The listing builds one solid part. Answer for the finished solid, in the listing's coordinates (mm). Coordinates: 2 decimals unless noted, no trailing zeros. Order: outer loops, then holes, each group sorted by start corner. A loop starts at its lowest first (then second) coordinate and runs counter-clockwise, first axis right, second up. Notation, with made-up numbers: (45, 43.5) -> (61, 43.5) arc R16 cw to (61, 57.5) -> close; hole circle Ø1 at (85.25, 7.25). An arc over 180 degrees is marked (long way). Return JSON: item names as keys, results as strings.
from build123d import *

# Parameters (mm, degrees)
BOSS_EXTRUDE1_DEPTH = 3
SKETCH2_R           = 3
CUT_EXTRUDE1_DEPTH  = 10
SKETCH3_R           = 3
CUT_EXTRUDE2_DEPTH  = 10


with BuildPart() as part:
    # Sketch1 → Boss-Extrude1 (new body)
    with BuildSketch(Plane.XY):
        with BuildLine():
            Line((0, 0), (170, 0))
            ThreePointArc((170, 0), (173.106601718, -7.5), (170, -15))
            Line((170, -15), (0, -15))
            ThreePointArc((0, -15), (-3.106601718, -7.5), (0, 0))
        make_face()
    extrude(amount=BOSS_EXTRUDE1_DEPTH)

    # Sketch2 → Cut-Extrude1 (cut)
    with BuildSketch(Plane.XY.offset(3)):
        with Locations((3, -7.5)):
            Circle(SKETCH2_R)
    extrude(amount=-CUT_EXTRUDE1_DEPTH, mode=Mode.SUBTRACT)

    # Sketch3 → Cut-Extrude2 (cut)
    with BuildSketch(Plane.XY.offset(3)):
        with Locations((167, -7.5)):
            Circle(SKETCH3_R)
    extrude(amount=-CUT_EXTRUDE2_DEPTH, mode=Mode.SUBTRACT)


solid = part.part
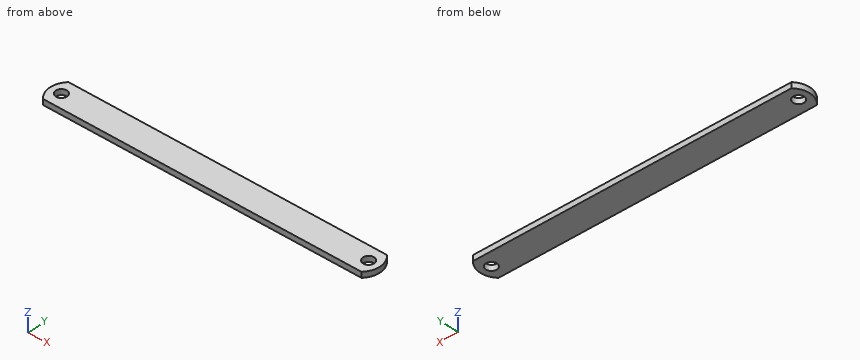
1. The part is cut by section A-A on x = 3. Give the vertices of the cut face in (y, z).
Answer block:
{"outline": "(-15, 0) -> (-10.5, 0) -> (-10.5, 3) -> (-15, 3) -> close; (-4.5, 0) -> (0, 0) -> (0, 3) -> (-4.5, 3) -> close"}
2. The part is cut by section C-C on z = 1.85. Give the vertices of the cut face in (x, y).
Answer block:
{"outline": "(0, -15) -> (170, -15) arc R10.61 ccw to (170, 0) -> (0, 0) arc R10.61 ccw to start; hole circle Ø6 at (3, -7.5); hole circle Ø6 at (167, -7.5)"}
3. Consider line 1 (Y direction, x = 3, z = 2.35); line 2 (X direction, y = -5, z = 2.45); line 3 (X direction, y = -7, z = 2). Determine where each line is inside the solid, lowest interval first. Write a range as from..to.
Answer block:
{"line 1": "y = -15..-10.5, -4.5..0", "line 2": "x = -2.81..1.34, 4.66..165.34, 168.66..172.81", "line 3": "x = -3.09..0.04, 5.96..164.04, 169.96..173.09"}
4. The part is cut by section B-B on y = -7.5. Give the vertices of the cut face in (x, z).
Answer block:
{"outline": "(-3.11, 0) -> (0, 0) -> (0, 3) -> (-3.11, 3) -> close; (6, 0) -> (164, 0) -> (164, 3) -> (6, 3) -> close; (170, 0) -> (173.11, 0) -> (173.11, 3) -> (170, 3) -> close"}
